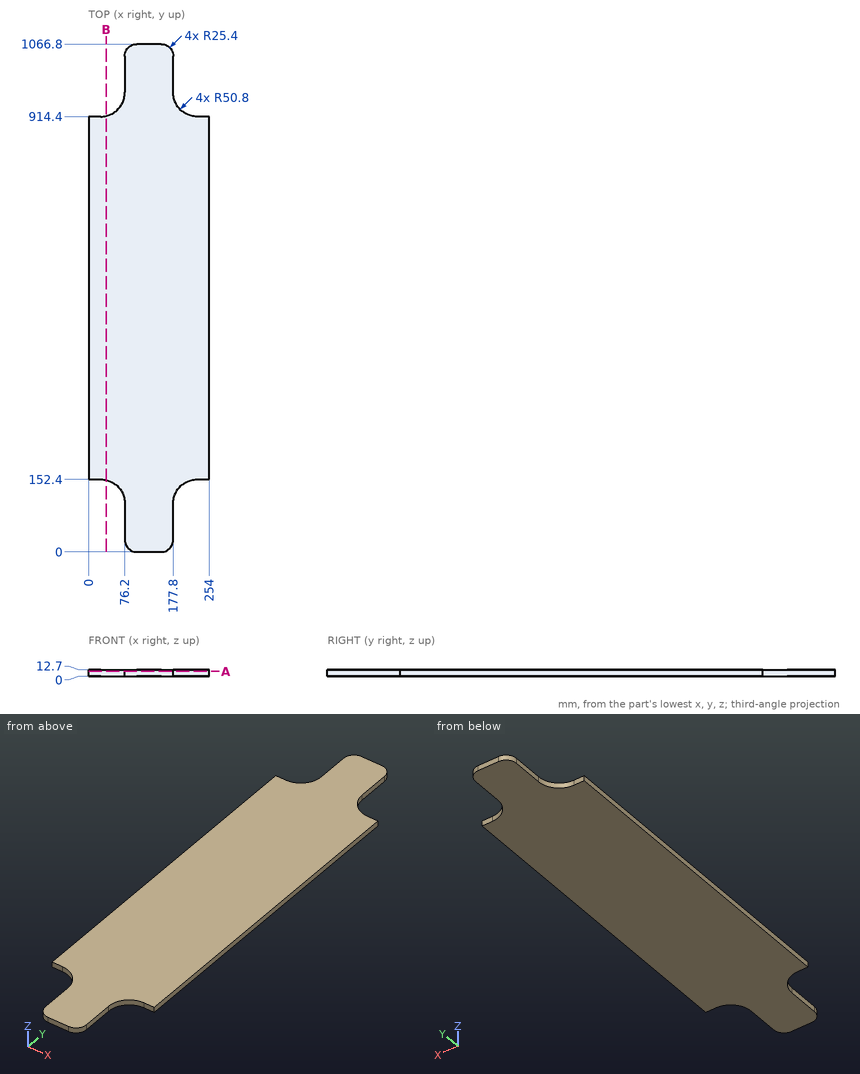
Check sheet for the drawn part. Datum: minimum x, y, z corner. Units: mm. Coordinates: 2 decimals unless noted, no trailing zeros. Loops run counter-clockwise (first coordinate to the right, second up) from the corner with the lowest first, then second, coordinate; pieces in that order, holes last. Notation, with made-up numbers: (88.25, 67.5) -> (114.25, 67.5) arc R13 cw to (114.25, 76.5) -> close; hole circle Ø4 at (66.25, 70.5). An arc over 180 degrees is marked (long way). Answer in a Markdown table with one row per item.
1. Material ranges on line 1 along Y through (x, z) = (230.5, 4.5); line 2 along Y through (x, z) = (99.5, 8); line 3 along X through (y, z) = (103.5, 12), recorded low to high. Write a range as [from, to].
Check values:
| item | result |
|---|---|
| line 1 | y = [152.4, 914.4] |
| line 2 | y = [0.09, 1066.71] |
| line 3 | x = [76.16, 177.84] |
2. Sectioned sample at B-B, the plane x = 37. Record the boundary of the cut face in (y, z).
Check values:
| item | result |
|---|---|
| outline | (151.06, 0) -> (915.74, 0) -> (915.74, 12.7) -> (151.06, 12.7) -> close |
3. Go/stop test with flat-tipped pins: pin 1 (1.5 mm diameter, centred on y = 122.5, z = 9, fed in from +X); pin 2 (10 mm diameter, centred on x = 56, y = 690, fed in from -Z); pin 3 (6.5 mm diameter, centred on x = 10, z = 8, fed in from +Y); pin 4 (4 mm diameter, centred on x = 14, z = 7, fed in from -Y). Record where each tip stops, or that it passes through.
Check values:
| item | result |
|---|---|
| pin 1 | stops at x = 182.64 |
| pin 2 | stops at z = 0 |
| pin 3 | stops at y = 914.4 |
| pin 4 | stops at y = 152.4 |
4. Sectioned sample at A-A, the plane z = 9.5. Record the boundary of the cut face in (x, y), then the cut area to 3 significant figures.
Check values:
| item | result |
|---|---|
| outline | (0, 152.4) -> (25.4, 152.4) arc R50.8 cw to (76.2, 101.6) -> (76.2, 25.4) arc R25.4 ccw to (101.6, 0) -> (152.4, 0) arc R25.4 ccw to (177.8, 25.4) -> (177.8, 101.6) arc R50.8 cw to (228.6, 152.4) -> (254, 152.4) -> (254, 914.4) -> (228.6, 914.4) arc R50.8 cw to (177.8, 965.2) -> (177.8, 1041.4) arc R25.4 ccw to (152.4, 1066.8) -> (101.6, 1066.8) arc R25.4 ccw to (76.2, 1041.4) -> (76.2, 965.2) arc R50.8 cw to (25.4, 914.4) -> (0, 914.4) -> close |
| area | 226,000 mm2 |
